Autodesk Inventor part; units mm, degrees
ref_plane "Work Plane1" through (-3.375, 19.5, 0) normal (0, 1, 0) x (1, 0, 0)
ref_plane "YZ Plane" through (0, 0, 0) normal (1, 0, 0) x (0, 1, 0)
ref_plane "XZ Plane" through (0, 0, 0) normal (0, 1, 0) x (-1, 0, 0)
sketch "Sketch2" plane through (0, 0, 0) normal (0, 0, 1) x (1, 0, 0)
  arc A0 (5, -12.1603) -> (-5, -12.1603) centre (0, -3.5) ccw
  line L0 (-5, -12.1603) -> (5, -12.1603) construction
  line L1 (5, -12.1603) -> (9.2376, -19.5)
  line L2 (-5, -12.1603) -> (-9.2376, -19.5)
  line L3 (-24, 8.5) -> (-22, 6.0385)
  line L4 (-22, 6.0385) -> (-22, -19.5)
  line L5 (24, 8.5) -> (22, 6.0385)
  line L6 (-22, -19.5) -> (-9.2376, -19.5)
  line L7 (22, 6.0385) -> (22, -19.5)
  line L8 (22, -19.5) -> (9.2376, -19.5)
  line L9 (-24, 17.5) -> (-22, 19.5)
  line L10 (-24, 17.5) -> (-24, 8.5)
  line L11 (24, 8.5) -> (24, 17.5)
  line L12 (24, 17.5) -> (22, 19.5)
  line L13 (-22, 19.5) -> (-14.125, 19.5)
  line L14 (-14.125, 19.5) -> (-13.125, 18.5)
  line L15 (-13.125, 18.5) -> (-4.375, 18.5)
  line L16 (-4.375, 18.5) -> (-3.375, 19.5)
  line L17 (-3.375, 19.5) -> (3.375, 19.5)
  line L18 (3.375, 19.5) -> (4.375, 18.5)
  line L19 (4.375, 18.5) -> (13.125, 18.5)
  line L20 (13.125, 18.5) -> (14.125, 19.5)
  line L21 (14.125, 19.5) -> (22, 19.5)
  point P0 (0, 0)
  point P1 (0, 0)
  point P2 (0, 0)
  dimension "h1" = 10
  dimension "r1" = 10
  dimension "d15" = 2
  dimension "d16" = 2
  dimension "d18" = 25.5385
  dimension "d19" = 25.5385
  dimension "d20" = 12.7624
  dimension "d21" = 12.7624
  dimension "d22" = 7.3398
  dimension "d23" = 7.3398
  dimension "d24" = 2.4615
  dimension "d25" = 2.4615
  dimension "d26" = 3.5
  dimension "d27" = 18.4752
  dimension "d28" = 22
  dimension "d33" = 2
  dimension "d34" = 2
  dimension "d35" = 9
  dimension "d36" = 2
  dimension "d37" = 44
  dimension "d38" = 9
  dimension "d40" = 1
  dimension "d41" = 8.75
  dimension "d42" = 8.75
  dimension "d43" = 6.75
  dimension "d44" = 1
  dimension "d45" = 1
  dimension "d46" = 1
  dimension "d47" = 7.875
  dimension "d48" = 7.875
extrude "Extrusion1" add sketch "Sketch2" along normal blind 50
ref_plane "Work Plane1" through (-3.375, 19.5, 0) normal (0, 1, 0) x (1, 0, 0)
sketch "Sketch3" plane through (-3.375, 19.5, 0) normal (0, 1, 0) x (1, 0, 0)
  line L0 (-20.625, 0) -> (3.375, 0) construction
  line L1 (-20.625, 0) -> (-20.625, -15.5497) construction
  line L2 (27.375, 0) -> (27.375, -50) construction
  line L3 (-18.625, 0) -> (-18.625, -50) construction
  line L4 (25.375, 0) -> (25.375, -50) construction
  point P0 (-14.125, -7.5)
  point P1 (20.875, -7.5)
  point P2 (-14.125, -42.5)
  point P3 (20.875, -42.5)
  dimension "d52" = 35
  dimension "d55" = 35
  dimension "d58" = 7.5
  dimension "d68" = 2
  dimension "d69" = 4.5
  dimension "d70" = 2
  dimension "d71" = 4.5
hole "Hole1" at (-17.5, 19.5, 7.5) at (17.5, 19.5, 7.5) at (-17.5, 19.5, 42.5) at (17.5, 19.5, 42.5) direction (0, -1, 0) diameter 6.3 depth 12 tip angle 118
equation "\"d16\" = d15"
equation "\"d19\" = d18"
equation "\"d21\" = d20"
equation "\"d23\" = d22"
equation "\"d25\" = d24"
equation "\"d34\" = d33"
equation "\"d42\" = d41"
equation "\"d44\" = d40"
equation "\"d45\" = d40"
equation "\"d46\" = d40"
equation "\"d48\" = d47"
properties part number "sbr20uu"
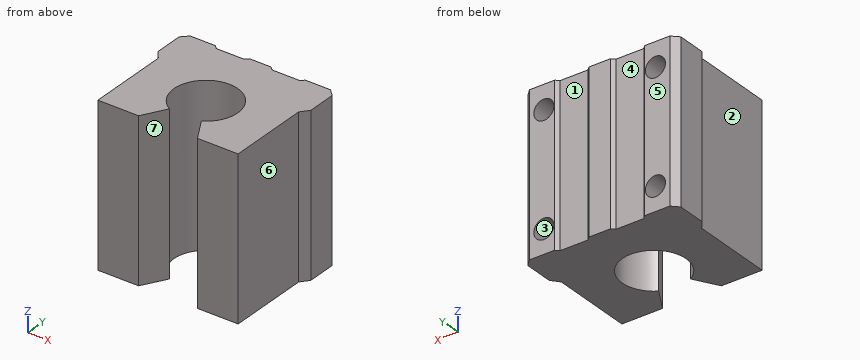
Can you work these out from the model? Positions are in its coordinate system, mm. Face numbers are marked on the shaded views. A direction names the side the tool comes from. Give positions to 0.01 mm unless a question says otherwise; leave off trailing zeros. Order: outer loops, then holes, each group sorted by start corner. A loop starts at its lowest first (then second) coordinate and runs counter-clockwise, first axis right, second up. Notation, with made-up numbers: M 69,29.25 L 125,29.25 A18 cw 125,49.25 Z; hole C 16.25,43.25 d3. An arc over 180 degrees is marked long. Use a Markdown table: item, result. Add a question column.
Item 1: Suppose I cut it at B-B (z = 20.5). List the corners of the cut face in (x, y) for me (1 decimal).
Item 2: Suppose I cut it at A-A (y = -3.5). List the corners of the cut face in (x, z) for me.
Item 3: Suppose I cut it at C-C (x = 6). List the corners of the cut face in (y, z) for me.
Item 4: Will these pins go through, and if not, where does the flat tip stop? pin 1 (5.5 mm diameter, centred on x = 17.5, z = 7.5, fed in from +Y); pin 2 (4 mm diameter, centred on x = -17.5, z = 7.5, fed in from +Y); pin 3 (7 mm diameter, centred on x = -9, z = 36.5, fed in from +Y).
Item 5: Suppose I cut it at D-D (y = 9.5). List the corners of the cut face in (x, z) for me.
Item 6: For the marked faces 1, 2 and 3, which set-ups out of +Z, -Z, +X, -X, +Y, -Y let a thin tool reach every point of the face, with its end or its side?
Item 7: If I drill on L1, parallel to Z at x = 17.5, y = 15.25; L2, parallel to X at y = 11, z = 42, over which ranges is the centre line in solid material (lowest first)? Write a range as [from, to].
Item 8: We'd pull the mould along X, two halves only. Please class the marked faces 4, 5, 6 and 7: +X half, -X half, draft (parallel to the pull), parting line (faces both ways), or undercut.
Answer sheet:
| question | item | result |
|---|---|---|
| 1 | outline | M -24,8.5 L -22,6 L -22,-19.5 L -9.2,-19.5 L -5,-12.2 A10 cw long 5,-12.2 L 9.2,-19.5 L 22,-19.5 L 22,6 L 24,8.5 L 24,17.5 L 22,19.5 L 14.1,19.5 L 13.1,18.5 L 4.4,18.5 L 3.4,19.5 L -3.4,19.5 L -4.4,18.5 L -13.1,18.5 L -14.1,19.5 L -22,19.5 L -24,17.5 Z |
| 2 | outline | M -22,0 L -10,0 L -10,50 L -22,50 Z; M 10,0 L 22,0 L 22,50 L 10,50 Z |
| 3 | outline | M -13.89,0 L -11.5,0 L -11.5,50 L -13.89,50 Z; M 4.5,0 L 18.5,0 L 18.5,50 L 4.5,50 Z |
| 4 | pin 1 | stops at y = 7.26 |
| 4 | pin 2 | stops at y = 6.81 |
| 4 | pin 3 | stops at y = 18.5 |
| 5 | outline | M -24,0 L 24,0 L 24,50 L -24,50 Z; hole C -17.5,7.5 d6.3; hole C -17.5,42.5 d6.3; hole C 17.5,7.5 d6.3; hole C 17.5,42.5 d6.3 |
| 6 | face 1 | +Z, -Z, +Y |
| 6 | face 2 | +Z, -Z, -X, -Y |
| 6 | face 3 | +Y |
| 7 | L1 | z = [0, 4.35], [10.65, 39.35], [45.65, 50] |
| 7 | L2 | x = [-24, -20.61], [-14.39, 14.39], [20.61, 24] |
| 8 | face 4 | undercut |
| 8 | face 5 | draft |
| 8 | face 6 | +X half |
| 8 | face 7 | undercut |
